Autodesk Inventor part; units mm, degrees
ref_plane "YZ Plane" through (0, 0, 0) normal (1, 0, 0) x (0, 1, 0)
ref_plane "XZ Plane" through (0, 0, 0) normal (0, 1, 0) x (-1, 0, 0)
ref_plane "XY Plane" through (0, 0, 0) normal (0, 0, 1) x (1, 0, 0)
sketch "Sketch1" plane through (0, 0, 0) normal (0, 0, 1) x (1, 0, 0)
  circle A0 centre (0, 0) radius 9
  line L0 (-3.4442, -8.3149) -> (3.4442, 8.3149) construction
  line L1 (-0.2106, -9.6543) -> (6.6777, 6.9755)
  line L2 (0.2106, 9.6543) -> (-6.6777, -6.9755)
  arc A1 (-6.6777, -6.9755) -> (-0.2106, -9.6543) centre (-3.4442, -8.3149) ccw
  arc A2 (6.6777, 6.9755) -> (0.2106, 9.6543) centre (3.4442, 8.3149) ccw
  line L3 (3.4442, -8.3149) -> (-3.4442, 8.3149) construction
  line L4 (6.6777, -6.9755) -> (-0.2106, 9.6543)
  line L5 (-6.6777, 6.9755) -> (0.2106, -9.6543)
  arc A3 (0.2106, -9.6543) -> (6.6777, -6.9755) centre (3.4442, -8.3149) ccw
  arc A4 (-0.2106, 9.6543) -> (-6.6777, 6.9755) centre (-3.4442, 8.3149) ccw
  line L6 (0, 0) -> (0, 9) construction
  dimension "d3" = 18
  dimension "d0" = 45
  dimension "d1" = 18
  dimension "d2" = 3.5
extrude "Extrusion1" add sketch "Sketch1" along normal blind 3
sketch "Sketch2" plane through (0, 0, 3) normal (0, 0, 1) x (1, 0, 0)
  arc A0 (-0.2106, 9.6543) -> (-6.6777, 6.9755) centre (-3.4442, 8.3149) ccw
  arc A1 (-6.6777, -6.9755) -> (-0.2106, -9.6543) centre (-3.4442, -8.3149) ccw
  arc A2 (0.2106, -9.6543) -> (6.6777, -6.9755) centre (3.4442, -8.3149) ccw
  arc A3 (6.4066, -6.321) -> (6.4066, 6.321) centre (0, 0) ccw
  arc A4 (6.6777, 6.9755) -> (0.2106, 9.6543) centre (3.4442, 8.3149) ccw
  circle A5 centre (-3.4442, 8.3149) radius 1.25
  circle A6 centre (3.4442, 8.3149) radius 1.25
  circle A7 centre (3.4442, -8.3149) radius 1.25
  circle A8 centre (-3.4442, -8.3149) radius 1.25
  circle A9 centre (0, 0) radius 6
  point P0 (0, 10.3491)
  point P1 (0, -10.3491)
  dimension "d6" = 2.5
  dimension "d7" = 12
extrude "Extrusion2" cut sketch "Sketch2" against normal through all
fillet "Fillet2" radius 1 2 edges at (0, -9.1459, 1.5) (0, 9.1459, 1.5)
sketch "Sketch3" plane through (0, 0, 3) normal (0, 0, 1) x (1, 0, 0)
  circle A0 centre (-3.4442, -8.3149) radius 1.25
  circle A1 centre (3.4442, 8.3149) radius 1.25
  circle A2 centre (-3.4442, 8.3149) radius 1.25
  circle A3 centre (3.4442, -8.3149) radius 1.25
  circle A4 centre (0, 0) radius 6
  arc A5 (-6.4066, 6.321) -> (-6.4066, -6.321) centre (0, 0) ccw
  line L0 (-6.4066, -6.321) -> (-6.6777, -6.9755)
  arc A6 (-6.6777, -6.9755) -> (-0.7654, -10.5675) centre (-3.4442, -8.3149) ccw
  arc A7 (0.7654, -10.5675) -> (-0.7654, -10.5675) centre (0, -11.2111) ccw
  arc A8 (0.7654, -10.5675) -> (6.6777, -6.9755) centre (3.4442, -8.3149) ccw
  line L1 (6.6777, -6.9755) -> (6.4066, -6.321)
  arc A9 (6.4066, -6.321) -> (6.4066, 6.321) centre (0, 0) ccw
  line L2 (6.4066, 6.321) -> (6.6777, 6.9755)
  arc A10 (6.6777, 6.9755) -> (0.7654, 10.5675) centre (3.4442, 8.3149) ccw
  arc A11 (-0.7654, 10.5675) -> (0.7654, 10.5675) centre (0, 11.2111) ccw
  arc A12 (-0.7654, 10.5675) -> (-6.6777, 6.9755) centre (-3.4442, 8.3149) ccw
  line L3 (-6.6777, 6.9755) -> (-6.4066, 6.321)
  circle A13 centre (-3.4442, -8.3149) radius 3 construction
  dimension "d12" = 6
properties part number "encoder_bearing_holder18_6mm_45"
Could you check a few things on this model? Use its own coordinates, in mm. Round coordinates to 2 decimals unless told otherwise and drop trailing zeros. Loops run counter-clockwise (first coordinate to the right, second up) from the corner with the lowest first, then second, coordinate; pieces in that order, holes last. Notation, with made-up numbers: (84, 31) -> (94, 31) arc R27 ccw to (94, 49) -> close; hole circle Ø5 at (-26, 88). An arc over 180 degrees is marked (long way). Put each result on its own line as item: value.
Q1. Thinking about a two-plate mould opening in Y: for faces 1 (the flat face through (-4, -5, 0)), 2 (the cylindrical face through (-6, 0, 2)), which applies, pulls with the +Y half, pulls with the -Y half, needs draft (parallel to the pull), parting line crosses it, or undercut?
Checks:
face 1: needs draft
face 2: undercut
Q2. I want a section at C-C on x = -5. Write out the boundary of the cut face in (y, z).
Checks:
outline: (-11.45, 0) -> (-3.32, 0) -> (-3.32, 3) -> (-11.45, 3) -> close; (3.32, 0) -> (11.45, 0) -> (11.45, 3) -> (3.32, 3) -> close
Q3. For pin 1 Ø1.5 at (x, z) = (5, 2) entering from +Y; pin 2 Ø1 at (y, z) = (3.5, 2) entering from -X; pin 3 Ø1 at (y, z) = (-2.5, 0.5) entering from -X, each with a flat end and sliding along its axis, tell me the tip position at first contact or that it passes through.
Checks:
pin 1: y = 11.72
pin 2: x = -8.49
pin 3: x = -8.77
Q4. Please list where these lines run through material, in increasing order: line 1 (X direction, y = 8.25, z = 1.75); line 2 (Y direction, x = 3.25, z = 1.65); line 3 (Y direction, x = 3.75, z = 2.5). Write a range as from..to.
Checks:
line 1: -6.94..-4.69, -2.2..2.2, 4.69..6.94
line 2: -11.81..-9.55, -7.08..-5.04, 5.04..7.08, 9.55..11.81
line 3: -11.8..-9.53, -7.1..-4.68, 4.68..7.1, 9.53..11.8
Q5. I want a section at D-D on x = 2.75. Write out the boundary of the cut face in (y, z), and give its area (3 significant figures).
Checks:
outline: (-11.75, 0) -> (-9.35, 0) -> (-9.35, 3) -> (-11.75, 3) -> close; (-7.28, 0) -> (-5.33, 0) -> (-5.33, 3) -> (-7.28, 3) -> close; (5.33, 0) -> (7.28, 0) -> (7.28, 3) -> (5.33, 3) -> close; (9.35, 0) -> (11.75, 0) -> (11.75, 3) -> (9.35, 3) -> close
area: 26.0 mm2
Q6. I want a section at A-A on y = 0. Write out the boundary of the cut face in (x, z), and give its area (3 significant figures).
Checks:
outline: (-9, 0) -> (-6, 0) -> (-6, 3) -> (-9, 3) -> close; (6, 0) -> (9, 0) -> (9, 3) -> (6, 3) -> close
area: 18.0 mm2
Q7. I want a section at B-B on y = -9. Write out the boundary of the cut face in (x, z), and give its area (3 significant figures).
Checks:
outline: (-6.88, 0) -> (-4.49, 0) -> (-4.49, 3) -> (-6.88, 3) -> close; (-2.4, 0) -> (2.4, 0) -> (2.4, 3) -> (-2.4, 3) -> close; (4.49, 0) -> (6.88, 0) -> (6.88, 3) -> (4.49, 3) -> close
area: 28.7 mm2
